```python
from build123d import *

# Parameters (mm, degrees)
BOSS_EXTRUDE1_DEPTH                                 = 14
FILLET1_R                                           = 10
FILLET2_R                                           = 60
SKETCH2_R                                           = 2.1
SKETCH2_R_2                                         = 3.062888277
CUT_EXTRUDE1_DEPTH                                  = 175.237067632
SKETCH3_R                                           = 2.5
CUT_EXTRUDE2_DEPTH                                  = 10
CBORE_FOR_M5_HEX_SOCKET_HEAD_CAP_SCREW1_D           = 5.5
CBORE_FOR_M5_HEX_SOCKET_HEAD_CAP_SCREW1_DEPTH       = 25
CBORE_FOR_M5_HEX_SOCKET_HEAD_CAP_SCREW1_CBORE_D     = 10
CBORE_FOR_M5_HEX_SOCKET_HEAD_CAP_SCREW1_CBORE_DEPTH = 8
CBORE_FOR_M5_HEX_SOCKET_HEAD_CAP_SCREW1_TIP         = 1.652366702
CUT_EXTRUDE3_DEPTH                                  = 25
FILLET3_R                                           = 10
CBORE_FOR_M5_HEX_SOCKET_HEAD_CAP_SCREW2_D           = 5.5
CBORE_FOR_M5_HEX_SOCKET_HEAD_CAP_SCREW2_DEPTH       = 25
CBORE_FOR_M5_HEX_SOCKET_HEAD_CAP_SCREW2_CBORE_D     = 10
CBORE_FOR_M5_HEX_SOCKET_HEAD_CAP_SCREW2_CBORE_DEPTH = 8
CBORE_FOR_M5_HEX_SOCKET_HEAD_CAP_SCREW2_TIP         = 1.652366702


with BuildPart() as part:
    # Sketch1 → Boss-Extrude1 (new body)
    with BuildSketch(Plane(origin=(0, 0, 0), x_dir=(1, 0, 0), z_dir=(0, 1, 0))):
        with BuildLine():
            Line((-68.874820235, 36.937111723), (-53.874820235, 36.937111723))
            Line((-53.874820235, 36.937111723), (-53.874820235, -43.062888277))
            Line((-53.874820235, -43.062888277), (-68.874820235, -43.062888277))
            ThreePointArc((-68.874820235, -43.062888277), (-97.683039558, -57.331289415), (-129.545963567, -53.058720487))
            Line((-129.545963567, -53.058720487), (-133.943104784, -59.313808797))
            ThreePointArc((-133.943104784, -59.313808797), (-147.874912369, -61.743775343), (-150.304878915, -47.811967758))
            Line((-150.304878915, -47.811967758), (-145.907737698, -41.556879448))
            ThreePointArc((-145.907737698, -41.556879448), (-161.623992411, -3.062888277), (-145.907737698, 35.431102894))
            Line((-145.907737698, 35.431102894), (-150.304878915, 41.686191203))
            ThreePointArc((-150.304878915, 41.686191203), (-147.874912369, 55.617998788), (-133.943104784, 53.188032242))
            Line((-133.943104784, 53.188032242), (-129.545963567, 46.932943933))
            ThreePointArc((-129.545963567, 46.932943933), (-97.683039558, 51.205512861), (-68.874820235, 36.937111723))
        make_face()
    extrude(amount=BOSS_EXTRUDE1_DEPTH)

    # Fillet1
    fillet1_edges = [part.edges().sort_by_distance(p)[0] for p in [
        (-53.874820235, 7, 43.062888277),
        (-129.545963567, 7, 53.058720487),
        (-145.907737698, 7, 41.556879448),
        (-129.545963567, 7, -46.932943933),
        (-53.874820235, 7, -36.937111723),
        (-145.907737698, 7, -35.431102894),
    ]]
    fillet(fillet1_edges, radius=FILLET1_R)

    # Fillet2
    fillet2_edges = [part.edges().sort_by_distance(p)[0] for p in [
        (-68.874820235, 7, 43.062888277),
        (-68.874820235, 7, -36.937111723),
    ]]
    fillet(fillet2_edges, radius=FILLET2_R)

    # Sketch2 → Cut-Extrude1 (cut, through all)
    with BuildSketch(Plane(origin=(0, 14, 0), x_dir=(1, 0, 0), z_dir=(0, 1, 0))):
        with Locations(Location((-106.623992411, 45.437111723, 0), (0, 0, 270))):
            Circle(SKETCH2_R)
        with Locations(Location((-72.329313524, 31.23179061, 0), (0, 0, 270))):
            Circle(SKETCH2_R)
        with Locations(Location((-58.123992411, -3.062888277, 0), (0, 0, 270))):
            Circle(SKETCH2_R)
        with Locations(Location((-72.329313524, -37.357567165, 0), (0, 0, 270))):
            Circle(SKETCH2_R)
        with Locations(Location((-106.623992411, -51.562888277, 0), (0, 0, 270))):
            Circle(SKETCH2_R)
        with Locations(Location((-140.918671299, -37.357567165, 0), (0, 0, 270))):
            Circle(SKETCH2_R)
        with Locations(Location((-155.123992411, -3.062888277, 0), (0, 0, 270))):
            Circle(SKETCH2_R)
        with Locations(Location((-140.918671299, 31.23179061, 0), (0, 0, 270))):
            Circle(SKETCH2_R)
        with Locations(Location((-106.623992411, -3.062888277, 0), (0, 0, 270))):
            Circle(SKETCH2_R_2)
    extrude(amount=-CUT_EXTRUDE1_DEPTH, mode=Mode.SUBTRACT)

    # Sketch3 → Cut-Extrude2 (cut)
    with BuildSketch(Plane(origin=(0, 14, 0), x_dir=(1, 0, 0), z_dir=(0, 1, 0))):
        with Locations(Location((-142.12399185, 47.437111723, 0), (0, 0, 270))):
            Circle(SKETCH3_R)
        with Locations(Location((-142.12399185, -53.562888277, 0), (0, 0, 270))):
            Circle(SKETCH3_R)
    extrude(amount=-CUT_EXTRUDE2_DEPTH, mode=Mode.SUBTRACT)

    # CBORE for M5 Hex Socket Head Cap Screw1
    with Locations(Plane(origin=(0, 14, 0), x_dir=(1, 0, 0), z_dir=(0, 1, 0))):
        with Locations((-89.123992411, 26.937111723), (-64.123992411, 26.937111723), (-76.623992411, -3.062888277), (-89.123992411, -33.062888277), (-64.123992411, -33.062888277)):
            CounterBoreHole(CBORE_FOR_M5_HEX_SOCKET_HEAD_CAP_SCREW1_D / 2, CBORE_FOR_M5_HEX_SOCKET_HEAD_CAP_SCREW1_CBORE_D / 2, CBORE_FOR_M5_HEX_SOCKET_HEAD_CAP_SCREW1_CBORE_DEPTH, depth=CBORE_FOR_M5_HEX_SOCKET_HEAD_CAP_SCREW1_DEPTH)
            with Locations((0, 0, -(CBORE_FOR_M5_HEX_SOCKET_HEAD_CAP_SCREW1_DEPTH + CBORE_FOR_M5_HEX_SOCKET_HEAD_CAP_SCREW1_TIP / 2))):  # 118° drill point
                Cone(0, CBORE_FOR_M5_HEX_SOCKET_HEAD_CAP_SCREW1_D / 2, CBORE_FOR_M5_HEX_SOCKET_HEAD_CAP_SCREW1_TIP, mode=Mode.SUBTRACT)

    # Sketch7 → Cut-Extrude3 (cut)
    with BuildSketch(Plane(origin=(0, 14, 0), x_dir=(1, 0, 0), z_dir=(0, 1, 0))):
        with BuildLine():
            Line((-98.692393489, -43.543158021), (-98.692393489, 37.417381467))
            ThreePointArc((-98.692393489, 37.417381467), (-147.873992411, -3.062888277), (-98.692393489, -43.543158021))
        make_face()
    extrude(amount=-CUT_EXTRUDE3_DEPTH, mode=Mode.SUBTRACT)

    # Fillet3
    fillet3_edges = [part.edges().sort_by_distance(p)[0] for p in [
        (-98.692393489, 7, 43.543158021),
        (-98.692393489, 7, -37.417381467),
    ]]
    fillet(fillet3_edges, radius=FILLET3_R)

    # CBORE for M5 Hex Socket Head Cap Screw2
    with Locations(Plane(origin=(0, 14, 0), x_dir=(1, 0, 0), z_dir=(0, 1, 0))):
        with Locations((-142.12399185, 47.437111723), (-142.12399185, -53.562888277)):
            CounterBoreHole(CBORE_FOR_M5_HEX_SOCKET_HEAD_CAP_SCREW2_D / 2, CBORE_FOR_M5_HEX_SOCKET_HEAD_CAP_SCREW2_CBORE_D / 2, CBORE_FOR_M5_HEX_SOCKET_HEAD_CAP_SCREW2_CBORE_DEPTH, depth=CBORE_FOR_M5_HEX_SOCKET_HEAD_CAP_SCREW2_DEPTH)
            with Locations((0, 0, -(CBORE_FOR_M5_HEX_SOCKET_HEAD_CAP_SCREW2_DEPTH + CBORE_FOR_M5_HEX_SOCKET_HEAD_CAP_SCREW2_TIP / 2))):  # 118° drill point
                Cone(0, CBORE_FOR_M5_HEX_SOCKET_HEAD_CAP_SCREW2_D / 2, CBORE_FOR_M5_HEX_SOCKET_HEAD_CAP_SCREW2_TIP, mode=Mode.SUBTRACT)


solid = part.part
```
Source: CAD feature listing. Evaluate the final solid. Frame: model axes, mm. A direction names the side the tool comes from. Round coordinates to 2 decimals unless told otherwise and drop trailing zeros. Write each loop counter-clockwise with the first axis right and the second up, starting at its lowest first coordinate (ties: lowest second). Pieces come first, ordered by that corner, then holes. Notation, with made-up numbers: M 85.5,16 L 122.5,16 A33 cw 122.5,54 Z; hole C 73,72.5 d10. An arc over 180 degrees is marked long. Answer as a JSON object with one key per item and string values. Group by question number.
(1) Reachability of faces 3 (the flat face through (-98.692, 7, 3)), 4 (the cylindrical face through (-99.261, 6.902, 57.568)), 5 (the flat face through (-140, 6, 56)) from +Z, -Z, +X, -X, +Y, -Y: full face, straight path, thin tool, end or side. Return the list, or none.
(2) First-contact query: pin 1 (5 mm diameter, centred on x = -65, z = -29, fed in from +Y); pin 2 (2 mm diameter, centred on x = -69, y = 10.5, fed in from +Z); pin 3 (6 mm diameter, centred on y = 10, z = 18.5, fed in from -X). Flat tips, straight axial feed; report the tip coordinate or a pass-through.
(3) Section query A-A on z = 23.5. Output: boundary loops of the cut face in (x, y).
(4) Section query C-C on y = 1.5. State how many separate pieces and enclosed holes the cut face has, then the cut area to 3 significant figures.
(5) Section query B-B on z = -13. Output: boundary loops of the cut face in (x, y), then the cut area to 3 significant figures.
(6) Mould query, pull axis X, two halves, no side actions, for faces 1 (the cylindrical face through (-104.54, 7.1, -45.71)), 2 (the cylindrical face through (-55.89, 7.1, 39.08)). Classes: +X half, -X half, draft (parallel to the pull), parting line (faces both ways), or undercut.
(7) Ray query, line 1 (Z direction, x = -92, y = 8.75); line 2 (X direction, y = 2.25, z = 32); line 3 (X direction, y = 10.75, z = 2.5). Return the intervals inside material, ascending. Write a range as [from, to].
Computed values:
{
 "1": {"face 3": "+Y, -Y", "face 4": "+Z, +Y, -Y", "face 5": "+Y"},
 "2": {"pin 1": "y = 6", "pin 2": "z = 45.77", "pin 3": "x = -160.2"},
 "3": {"outline": "M -157.69,0 L -142.46,0 L -142.46,14 L -157.69,14 Z; M -98.69,0 L -53.87,0 L -53.87,14 L -98.69,14 Z"},
 "4": {"separate pieces": "1", "enclosed holes": "16", "area": "6,810 mm^2"},
 "5": {"outline": "M -159.23,0 L -144.62,0 L -144.62,14 L -159.23,14 Z; M -98.69,0 L -53.87,0 L -53.87,14 L -98.69,14 Z", "area": "832 mm^2"},
 "6": {"face 1": "undercut", "face 2": "+X half"},
 "7": {"line 1": "[-49.96, -31.03], [-22.85, 28.97], [37.15, 56.08]", "line 2": "[-153.4, -136.02], [-98.69, -91.66], [-86.59, -66.66], [-61.59, -53.87]", "line 3": "[-161.62, -157.15], [-153.1, -147.87], [-98.69, -81.59], [-71.66, -60.15], [-56.1, -53.87]"}
}
